The model under review builds one solid part; all positions refer to its coordinate system, in mm. A direction names the side the tool comes from. Give positions to 0.01 mm unless a question says otherwise; leave off trailing zeros. Loops run counter-clockwise (first coordinate to the right, second up) from the corner with the lowest first, then second, coordinate; pieces in that order, holes last. Notation, with made-up numbers: M 34.5,72.25 L 50.5,72.25 A3 ccw 50.5,76.25 Z; hole C -27.5,3 d9. An arc over 180 degrees is marked long. Write item = value, one per line. Start each with the question number.
1. We need section C-C on x = -2.3. Give the boundary of the cut face in (y, z), then the cut area to 3 significant figures.
2. For faces 1 (the face through (-0.749, 2.169, 1.184)), 2 (the face through (-1, 2, 2.05)), list the 3-axis set-ups (+Z, -Z, +X, -X, +Y, -Y) from which the entire face can be reached by the end or side of a thin tool; tool diameter is ignored.
3. Draft analysis for pull direction Z (two halves, no side actions). For faces 3 (the face through (-1.5, 0, 0.9)), 4 (the face through (-1, 2, -2.05)), 5 (the face through (-2.146, 2.5, 0.954)), state which applies: pulls with the +Z half, pulls with the -Z half, needs draft (parallel to the pull), parting line crosses it, or undercut.
4. For pin 1 (2 mm diameter, centred on x = 0, z = 0, fed in from +Y); pin 2 (1 mm diameter, centred on y = 2.5, z = -0.5, fed in from +X); pin 3 (1.6 mm diameter, centred on y = 2.2, z = 0, fed in from -X), all flat-tipped, find the tip position at first contact; note any pin that passes through.
5. We need section D-D on y = 2.2. Give the boundary of the cut face in (x, z).
6. Wall thickness on line 1 along Z through (x, y) = (-0.15, 3); line 2 along Y through (x, z) = (-2.3, 0); line 3 along Z through (x, y) = (-1.8, 2.2): over which ranges is each line inside the solid? List them lowest first. Write a range as from..to.
7. We need section A-A on x = -0.2. Give the boundary of the cut face in (y, z), then the cut area to 3 significant figures.
8. We need section B-B on y = 0.8. Give the boundary of the cut face in (x, z).
Autodesk Inventor part; units mm, degrees
ref_plane "YZ Plane" through (0, 0, 0) normal (1, 0, 0) x (0, 1, 0)
ref_plane "XZ Plane" through (0, 0, 0) normal (0, 1, 0) x (-1, 0, 0)
ref_plane "XY Plane" through (0, 0, 0) normal (0, 0, 1) x (1, 0, 0)
sketch "Sketch1" plane through (0, 0, 0) normal (0, 1, 0) x (-1, 0, 0)
  circle A0 centre (-0.4, 0) radius 2.05
  line L0 (-0.4, 2.05) -> (3.05, 2.05)
  line L1 (3.05, 2.05) -> (3.05, -2.05)
  line L2 (3.05, -2.05) -> (-0.4, -2.05)
  line L3 (-2.45, 0) -> (-2.45, -1.163)
  line L4 (-1.45, 0) -> (1.45, 0) construction
  line L5 (-0.1, -1.35) -> (0.1, -1.35)
  line L6 (0.1, 1.35) -> (-0.1, 1.35)
  arc A1 (-0.1, 1.35) -> (-0.1, -1.35) centre (-0.1, 0) ccw
  arc A2 (0.1, -1.35) -> (0.1, 1.35) centre (0.1, 0) ccw
  point P0 (0, 0)
  point P1 (0, 0)
  dimension "d1" = 4.1
  dimension "d2" = 5.5
  dimension "d3" = 2.7
  dimension "d4" = 2.9
  dimension "d5" = 1
extrude "Extrusion1" add sketch "Sketch1" along normal blind 4.4
sketch "Sketch2" plane through (-3.05, 0, -2.05) normal (-1, 0, 0) x (0, 0, 1)
  line L0 (0, 0) -> (4.1, 0)
  line L1 (4.1, 0) -> (4.1, 4.4)
  line L2 (0, 4.4) -> (4.1, 4.4)
  line L3 (0, 0) -> (0, 4.4)
  circle A0 centre (2.05, 2.2) radius 1
  point P0 (2.05, 0)
  dimension "d8" = 2
extrude "Extrusion2" cut sketch "Sketch2" against normal up to surface contours A0
thread "Thread1"
chamfer "Chamfer1" distance 0.2 angle 45 1 edges at (-3.05, 2.2, -1)
properties part number "metal_connector" material "Steel, Alloy"
Final values:
q1.outline = M 0,-2.05 L 4.4,-2.05 L 4.4,2.05 L 0,2.05 Z; hole C 2.2,0 d2
q1.area = 14.9 mm²
q2.face_1 = +Y, -Y
q2.face_2 = +Z, +X, -X, +Y, -Y
q3.face_3 = needs draft
q3.face_4 = pulls with the -Z half
q3.face_5 = undercut
q4.pin_1 = through
q4.pin_2 = 2.45
q4.pin_3 = 1.19
q5.outline = M -3.05,-2.05 L 0.4,-2.05 A2.05 ccw 0.4,2.05 L -3.05,2.05 L -3.05,1.2 L -2.85,1 L -1.01,1 A1.35 cw -0.1,1.35 L 0.1,1.35 A1.35 cw 0.1,-1.35 L -0.1,-1.35 A1.35 cw -1.01,-1 L -2.85,-1 L -3.05,-1.2 Z
q6.line_1 = -2.05..-1.35, 1.35..2.05
q6.line_2 = 0..1.2, 3.2..4.4
q6.line_3 = -2.05..-1, 1..2.05
q7.outline = M 0,-2.05 L 4.4,-2.05 L 4.4,-1.35 L 0,-1.35 Z; M 0,1.35 L 4.4,1.35 L 4.4,2.05 L 0,2.05 Z
q7.area = 6.19 mm²
q8.outline = M -3.05,-2.05 L 0.4,-2.05 A2.05 ccw 0.4,2.05 L -3.05,2.05 Z; hole M -0.1,-1.35 L 0.1,-1.35 A1.35 ccw 0.1,1.35 L -0.1,1.35 A1.35 ccw Z
